Geometry check sheet. Reference: the model listing, model coordinates, mm. A direction names the side the tool comes from. Coordinates: 2 decimals unless noted, no trailing zeros. Loops run counter-clockwise (first coordinate to the right, second up) from the corner with the lowest first, then second, coordinate; pieces in that order, holes last.
from build123d import *

# Parameters (mm, degrees)
BOSS_EXTRUDE1_DEPTH = 12.7
BOSS_EXTRUDE2_REACH = 70.373
SKETCH4_W           = 12.7
SKETCH4_H           = 34.6329
SKETCH6_W           = 3.175
SKETCH6_H           = 8.382
BOSS_EXTRUDE3_DEPTH = 19.05
SKETCH7_R           = 2.1828125
CUT_EXTRUDE1_DEPTH  = 12.7


with BuildPart() as part:
    # Sketch1 → Boss-Extrude1 (new body)
    with BuildSketch(Plane(origin=(0, 0, 0), x_dir=(0, 0, -1), z_dir=(1, 0, 0))):
        with BuildLine():
            Line((28.295148135, 2.354226963), (52.253698135, 2.354226963))
            Line((52.253698135, 2.354226963), (52.253698135, 8.704226963))
            Line((52.253698135, 8.704226963), (31.470148135, 8.704226963))
            Line((31.470148135, 8.704226963), (31.470148135, 16.495676963))
            ThreePointArc((31.470148135, 16.495676963), (14.153698135, 33.812126963), (-3.162751865, 16.495676963))
            Line((-3.162751865, 16.495676963), (-3.162751865, 8.704226963))
            Line((-3.162751865, 8.704226963), (-23.946301865, 8.704226963))
            Line((-23.946301865, 8.704226963), (-23.946301865, 2.354226963))
            Line((-23.946301865, 2.354226963), (0.012248135, 2.354226963))
            Line((0.012248135, 2.354226963), (0.012248135, 16.495676963))
            ThreePointArc((0.012248135, 16.495676963), (14.153698135, 30.637126963), (28.295148135, 16.495676963))
            Line((28.295148135, 16.495676963), (28.295148135, 2.354226963))
        make_face()
    extrude(amount=BOSS_EXTRUDE1_DEPTH)

    # Sketch4 → Boss-Extrude2 (add, up to next)
    with BuildSketch(Plane(origin=(0, 44.581726963, 0), x_dir=(1, 0, 0), z_dir=(0, 1, 0)), mode=Mode.PRIVATE) as boss_extrude2_sk1:
        with Locations((6.35, 14.153698135)):
            Rectangle(SKETCH4_W, SKETCH4_H)
    boss_extrude2_tool1 = extrude(boss_extrude2_sk1.sketch, amount=-BOSS_EXTRUDE2_REACH, mode=Mode.PRIVATE) - part.part
    add(boss_extrude2_tool1.solids().sort_by_distance((6.35, 44.581727, -14.153698))[0])

    # Sketch6 → Boss-Extrude3 (add)
    with BuildSketch(Plane(origin=(12.7, 0, 0), x_dir=(0, 0, -1), z_dir=(1, 0, 0))):
        with Locations((-1.784801865, 40.390726963)):
            Rectangle(SKETCH6_W, SKETCH6_H)
        with Locations((30.092198135, 40.390726963)):
            Rectangle(SKETCH6_W, SKETCH6_H)
    extrude(amount=BOSS_EXTRUDE3_DEPTH)

    # Sketch7 → Cut-Extrude1 (cut)
    with BuildSketch(Plane(origin=(0, 8.704226963, 0), x_dir=(1, 0, 0), z_dir=(0, 1, 0))):
        with Locations(Location((6.35, 41.861923135, 0), (0, 0, 270))):
            Circle(SKETCH7_R)
        with Locations(Location((6.35, -13.554526865, 0), (0, 0, 270))):
            Circle(SKETCH7_R)
    extrude(amount=-CUT_EXTRUDE1_DEPTH, mode=Mode.SUBTRACT)

    # Mirror1: part across plane


with BuildPart() as part_1:
    add(part.part)
    add(part.part.mirror(Plane(origin=(31.75, 0, 0), x_dir=(0, 0, 1), z_dir=(1, 0, 0))))


solid = part_1.part
1) Section check B-B on z = 9. Record the cut outline in (x, y).
Data:
outline: (0, 2.35) - (12.7, 2.35) - (12.7, 8.7) - (0, 8.7) - close; (50.8, 2.35) - (63.5, 2.35) - (63.5, 8.7) - (50.8, 8.7) - close
2) Section check A-A on y = 7.5. Record the cut outline in (x, z), and give its area (3 significant figures).
Data:
outline: (0, -52.25) - (12.7, -52.25) - (12.7, -28.3) - (0, -28.3) - close; (0, -0.01) - (12.7, -0.01) - (12.7, 23.95) - (0, 23.95) - close; (50.8, -52.25) - (63.5, -52.25) - (63.5, -28.3) - (50.8, -28.3) - close; (50.8, -0.01) - (63.5, -0.01) - (63.5, 23.95) - (50.8, 23.95) - close; hole circle Ø4.37 at (6.35, -41.86); hole circle Ø4.37 at (6.35, 13.55); hole circle Ø4.37 at (57.15, -41.86); hole circle Ø4.37 at (57.15, 13.55)
area: 1,160 mm2
3) Mould release check, pull along X, two halves, no side actions. Record for faces 4 (the flat face through (0, 31, -11)), 5 (the flat face through (57, 9, -0.012)), 6 (the flat face through (63.5, 31, -11)), 7 (the flat face through (32, 36.2, -30)): +X half, -X half, draft (parallel to the pull), parting line (faces both ways), or undercut.
Data:
face 4: -X half
face 5: draft
face 6: +X half
face 7: undercut
4) Section check C-C on x = 6.35. Record the cut outline in (y, z), and give its area (3 significant figures).
Data:
outline: (2.35, -52.25) - (8.7, -52.25) - (8.7, -44.04) - (2.35, -44.04) - close; (2.35, -39.68) - (8.7, -39.68) - (8.7, -31.47) - (44.58, -31.47) - (44.58, 3.16) - (8.7, 3.16) - (8.7, 11.37) - (2.35, 11.37) - (2.35, -0.01) - (16.5, -0.01) arc R14.14 cw to (16.5, -28.3) - (2.35, -28.3) - close; (2.35, 15.74) - (8.7, 15.74) - (8.7, 23.95) - (2.35, 23.95) - close
area: 957 mm2
5) Section check D-D on x = 46.5. Record the cut outline in (y, z), and give its area (3 significant figures).
Data:
outline: (36.2, -31.68) - (44.58, -31.68) - (44.58, -28.5) - (36.2, -28.5) - close; (36.2, 0.2) - (44.58, 0.2) - (44.58, 3.37) - (36.2, 3.37) - close
area: 53.2 mm2
6) Material ranges on probe 1 along Z at (x, y) = (57.15, 5.5); probe 2 along X at (y, z) = (10.5, 0.5); probe 3 along Z at (x, y) = (49, 37), recorded low to high.
Data:
probe 1: z = -52.25 to -44.04, -39.68 to -28.3, -0.01 to 11.37, 15.74 to 23.95
probe 2: x = 0 to 12.7, 50.8 to 63.5
probe 3: z = -31.68 to -28.5, 0.2 to 3.37
7) Depth check by flat-ended pin: pin 1 (2.5 mm diameter, centred on x = 24, y = 39, fed in from +Z); pin 2 (6 mm diameter, centred on x = 30.5, z = -0.5, fed in from -Y); pin 3 (12 mm diameter, centred on x = 53, z = 10.5, fed in from +Y); pin 4 (3.5 mm diameter, centred on x = 6.35, z = 13.55, fed in from +Y). Enter the tip coordinate at first touch or a pass-through.
Data:
pin 1: stops at z = 3.37
pin 2: stops at y = 36.2
pin 3: stops at y = 8.7
pin 4: passes through
8) Access from +Z, -Z, +X, -X, +Y, -Y to the whole of each face (thin tool, end or side, straight path). Record for faces 1 (the flat face through (57, 8.704, 11)), 2 (the flat face through (57, 27, 3.163)), 3 (the flat face through (6, 9, -0.012)).
Data:
face 1: +Z, +X, -X, +Y
face 2: +Z, +X, +Y
face 3: +X, -X, -Y
